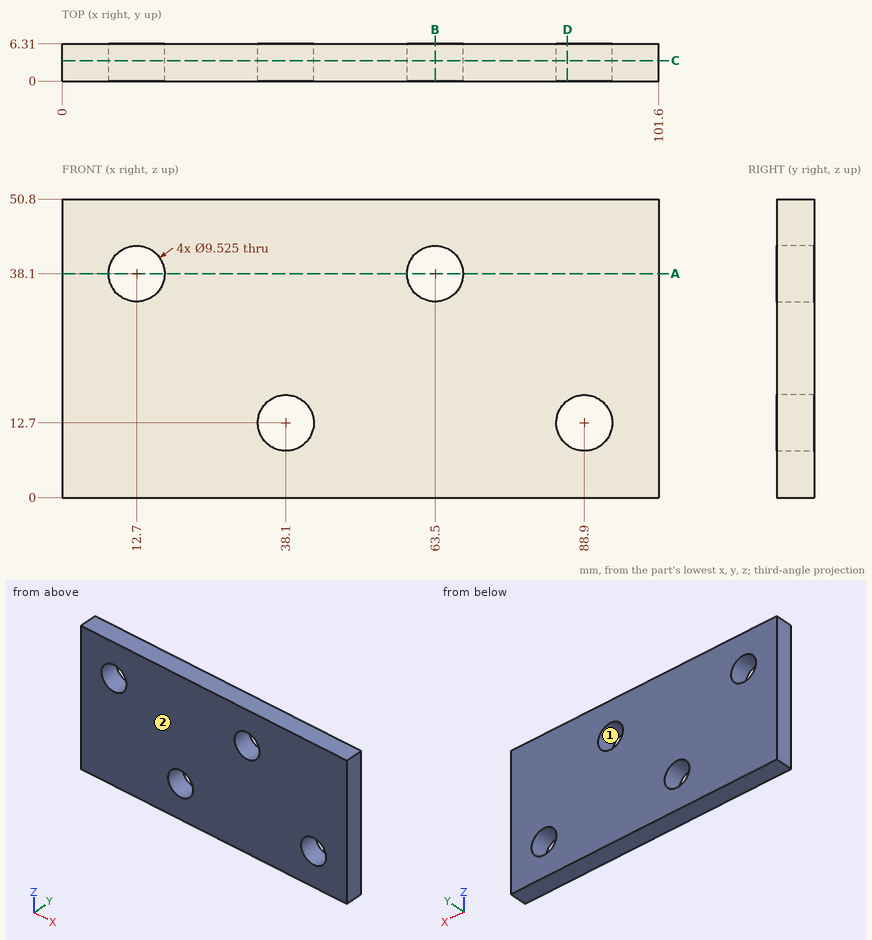
Check sheet for the drawn part. Datum: minimum x, y, z corner. Units: mm. Round coordinates to 2 decimals unless told otherwise and drop trailing zeros. Order: outer loops, then holes, each group sorted by start corner. A loop starts at its lowest first (then second) coordinate and runs counter-clockwise, first axis right, second up. Notation, with made-up numbers: M -1.75,-15 L 7.25,-15 A21 cw 7.25,23 Z; hole C 65.25,44.5 d11. An arc over 180 degrees is marked long. Write each question's results on one line, items separated by ' | '. Start each with the question number.
1. Draft check along X on the marked faces 1 and 2. Enter one of: pulls with the +X half, pulls with the -X half, needs draft (parallel to the pull), parting line crosses it, or undercut.
2. Cross-section at D-D on x = 86. Record the boundary of the cut face in (y, z), plus the area to 3 significant figures.
3. Material ranges on L1, parallel to X at y = 3.75, z = 38.1; L2, parallel to X at y = 1.5, z = 12.7; L3, parallel to Z at x = 88.9, y = 3.25, recorded low to high. Write a range as from..to.
4. Cross-section at A-A on z = 38.1. Record the boundary of the cut face in (x, y), plus the area to 3 significant figures.
5. Cross-section at B-B on x = 63.5. Record the boundary of the cut face in (y, z), plus the area to 3 significant figures.
6. Cross-section at C-C on y = 3.5. Record the boundary of the cut face in (x, z) (1 decimal), plus the area to 3 significant figures.
Resolved:
1) face 1: undercut | face 2: needs draft
2) outline: M 0,0 L 6.31,0 L 6.31,8.92 L 0,8.92 Z; M 0,16.48 L 6.31,16.48 L 6.31,50.8 L 0,50.8 Z | area: 273 mm2
3) L1: 0..7.94, 17.46..58.74, 68.26..101.6 | L2: 0..33.34, 42.86..84.14, 93.66..101.6 | L3: 0..7.94, 17.46..50.8
4) outline: M 0,0 L 7.94,0 L 7.94,6.31 L 0,6.31 Z; M 17.46,0 L 58.74,0 L 58.74,6.31 L 17.46,6.31 Z; M 68.26,0 L 101.6,0 L 101.6,6.31 L 68.26,6.31 Z | area: 521 mm2
5) outline: M 0,0 L 6.31,0 L 6.31,33.34 L 0,33.34 Z; M 0,42.86 L 6.31,42.86 L 6.31,50.8 L 0,50.8 Z | area: 260 mm2
6) outline: M 0,0 L 101.6,0 L 101.6,50.8 L 0,50.8 Z; hole C 12.7,38.1 d9.5; hole C 38.1,12.7 d9.5; hole C 63.5,38.1 d9.5; hole C 88.9,12.7 d9.5 | area: 4,880 mm2
